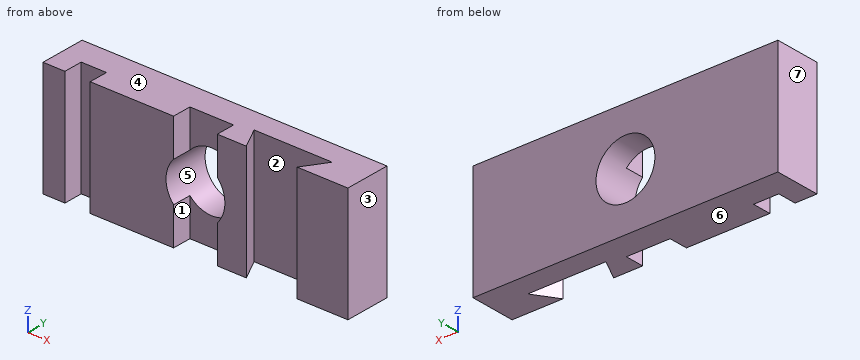
```python
from build123d import *

# Parameters (mm, degrees)
F0_W     = 203.2
F0_H     = 76.2
F1_DEPTH = 30.48
F2_R     = 19.62516
F3_DEPTH = 30.481
F4_W     = 16.807922
F4_H     = 76.2
F4_W_2   = 29.126016
F5_DEPTH = 12.7
F7_DEPTH = 76.201


with BuildPart() as f1:
    # F0 (on Front) → F1 (new body)
    with BuildSketch(Plane.XZ):
        Rectangle(F0_W, F0_H)
    extrude(amount=F1_DEPTH)

    # F2 (on face) → F3 (cut, through all)
    with BuildSketch(Plane.XZ.offset(30.48)):
        Circle(F2_R)
    extrude(amount=-F3_DEPTH, mode=Mode.SUBTRACT)

    # F4 (on face) → F5 (cut)
    with BuildSketch(Plane.XZ.offset(30.48)):
        with Locations((-78.576129, 0)):
            Rectangle(F4_W, F4_H)
        Rectangle(F4_W_2, F4_H)
    extrude(amount=-F5_DEPTH, mode=Mode.SUBTRACT)

    # F6 (on face) → F7 (cut, through all)
    with BuildSketch(Plane(origin=(0, 0, -38.1), x_dir=(1, 0, 0), z_dir=(0, 0, -1))):
        Polygon((67.76917, 30.48), (33.899248, 30.48), (25.846235, 14.998903), (77.894919, 14.998903), align=None)
    extrude(amount=-F7_DEPTH, mode=Mode.SUBTRACT)


solid = f1.part
```
Source: CAD feature listing. Evaluate the final solid. Frame: model axes, mm. Face numbers are marked on the shaded views. A direction names the side the tool comes from. Give positions to 0.01 mm unless a question says otherwise; leave off trailing zeros. Loops run counter-clockwise (first coordinate to the right, second up) from the corner with the lowest first, then second, coordinate; pieces in that order, holes last. Notation, with made-up numbers: M 73.5,58 L 127.5,58 A34 cw 127.5,91 Z; hole C 17,16.5 d2. An arc over 180 degrees is marked long. Put each result on its own line as item: value.
Q1. Mould query, pull axis Z, two halves, no side actions, for the marked faces 4, 5, 6 and 7. Classes: released by +Z, released by -Z, zero draft, split by the parting line, or undercut.
Response values:
face 4: released by +Z
face 5: undercut
face 6: released by -Z
face 7: zero draft
Q2. Pin query (flat end, axial travel): P1, Ø3, axis at x = 41, y = -17, coming from the -Z side; P2, Ø7.5, axis at x = -4, z = 23, coming from the -Y side. Return the tip coordinate at first contact, or that it passes through.
Response values:
P1: passes through
P2: stops at y = -17.78
Q3. Section A-A (x = 0). Return the cut outline in (y, z), and give its area (3 significant figures).
Response values:
outline: M -17.78,-38.1 L 0,-38.1 L 0,-19.63 L -17.78,-19.63 Z; M -17.78,19.63 L 0,19.63 L 0,38.1 L -17.78,38.1 Z
area: 657 mm²
Q4. Line query: probe 1 along X at (y, z) = (-11, 0); probe 2 along Z at (x, y) = (0, -12.5); probe 3 along X at (y, z) = (-26, 2). Output: solid intervals per line, ascending. Write a range as [from, to].
Response values:
probe 1: x = [-101.6, -19.63], [19.63, 101.6]
probe 2: z = [-38.1, -19.63], [19.63, 38.1]
probe 3: x = [-101.6, -86.98], [-70.17, -19.52], [19.52, 31.57], [70.7, 101.6]
Q5. Reachability of the marked faces 1, 2 and 3 from +Z, -Z, +X, -X, +Y, -Y: full face, straight path, thin tool, end or side. Return the list, or none.
Response values:
face 1: +Z, -Z, -Y
face 2: +Z, -Z
face 3: +Z, -Z, +X, +Y, -Y
Q6. Section B-B (z = 0). Return the cut outline in (x, y).
Response values:
outline: M -101.6,-30.48 L -86.98,-30.48 L -86.98,-17.78 L -70.17,-17.78 L -70.17,-30.48 L -19.63,-30.48 L -19.63,0 L -101.6,0 Z; M 19.63,-30.48 L 33.9,-30.48 L 25.85,-15 L 77.89,-15 L 67.77,-30.48 L 101.6,-30.48 L 101.6,0 L 19.63,0 Z
Q7. Section D-D (y = -13). Return the cut outline in (x, z), and give its area (3 significant figures).
Response values:
outline: M -101.6,-38.1 L 101.6,-38.1 L 101.6,38.1 L -101.6,38.1 Z; hole C 0,0 d39.25
area: 14,300 mm²
Q8. Section C-C (y = -27.5). Return the cut outline in (x, z), and give its area (3 significant figures).
Response values:
outline: M -101.6,-38.1 L -86.98,-38.1 L -86.98,38.1 L -101.6,38.1 Z; M -70.17,-38.1 L -14.56,-38.1 L -14.56,-13.16 A19.63 cw -14.56,13.16 L -14.56,38.1 L -70.17,38.1 Z; M 14.56,-38.1 L 32.35,-38.1 L 32.35,38.1 L 14.56,38.1 L 14.56,13.16 A19.63 cw 14.56,-13.16 Z; M 69.72,-38.1 L 101.6,-38.1 L 101.6,38.1 L 69.72,38.1 Z
area: 8,950 mm²
